Geometry check sheet. Reference: the model listing, model coordinates, mm. Face numbers are marked on the shaded views. A direction names the side the tool comes from. Give positions to 0.01 mm unless a question says otherwise; leave off trailing zeros. Use CSV: the item, a comma, the result in double quotes. Start each with the question number.
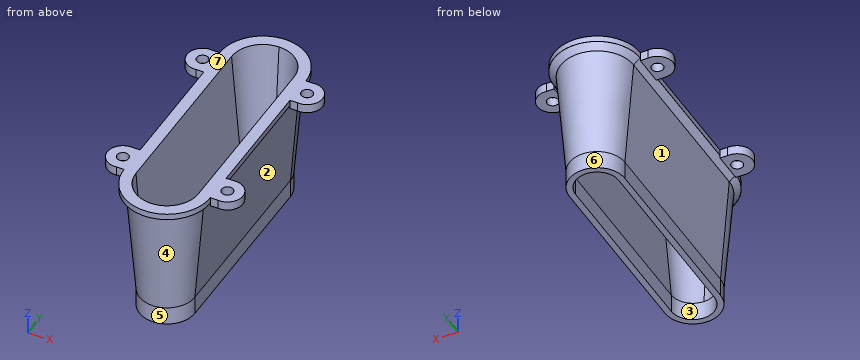
from build123d import *
from OCP.BRepFilletAPI import BRepFilletAPI_MakeChamfer

# Parameters (mm, degrees)
DODANIE_WYCI_GNI_CIE1_DEPTH  = 45
DODANIE_WYCI_GNI_CIE2_DEPTH  = 2
SFAZOWANIE1_SIZE             = 37
SFAZOWANIE1_SIZE2            = 3
SKORUPA4_DEPTH               = 45
SZKIC11_R                    = 1.9
DODANIE_WYCI_GNI_CIE11_DEPTH = 3
SFAZOWANIE6_SIZE             = 1.8
SFAZOWANIE6_SIZE2            = 1.965251773


with BuildPart() as part:
    # Szkic1 → Dodanie-wyciągnięcie1 (new body)
    with BuildSketch(Plane.XY):
        with BuildLine():
            Line((-9, 0), (-9, 60))
            ThreePointArc((-9, 60), (0, 69), (9, 60))
            Line((9, 60), (9, 0))
            ThreePointArc((9, 0), (0, -9), (-9, 0))
        make_face()
    extrude(amount=DODANIE_WYCI_GNI_CIE1_DEPTH)

    # Szkic2 → Dodanie-wyciągnięcie2 (add)
    with BuildSketch(Plane.XY.offset(45)):
        with BuildLine():
            Line((14, 60), (14, 0))
            ThreePointArc((14, 0), (0, -14), (-14, 0))
            Line((-14, 0), (-14, 60))
            ThreePointArc((-14, 60), (0, 74), (14, 60))
        make_face()
    extrude(amount=-DODANIE_WYCI_GNI_CIE2_DEPTH)

    # Sfazowanie1: one chamfer whose edges measure the first distance from different faces: ONE call of the kernel's chamfer builder (chamfer() names one face for all edges)
    sfazowanie1_edges_1 = [part.edges().sort_by_distance(p)[0] for p in [
        (-9, 30, 43),
    ]]
    sfazowanie1_side_1 = [part.faces().sort_by_distance(p)[0] for p in [
        (-9, 30, 21.5),
    ]]
    sfazowanie1_edges_2 = [part.edges().sort_by_distance(p)[0] for p in [
        (0, -9, 43),
    ]]
    sfazowanie1_side_2 = [part.faces().sort_by_distance(p)[0] for p in [
        (0, -9, 21.5),
    ]]
    sfazowanie1_edges_3 = [part.edges().sort_by_distance(p)[0] for p in [
        (9, 30, 43),
    ]]
    sfazowanie1_side_3 = [part.faces().sort_by_distance(p)[0] for p in [
        (9, 30, 21.5),
    ]]
    sfazowanie1_edges_4 = [part.edges().sort_by_distance(p)[0] for p in [
        (0, 69, 43),
    ]]
    sfazowanie1_side_4 = [part.faces().sort_by_distance(p)[0] for p in [
        (0, 69, 21.5),
    ]]
    sfazowanie1 = BRepFilletAPI_MakeChamfer(part.part.solid().wrapped)
    for e in sfazowanie1_edges_1:
        sfazowanie1.Add(SFAZOWANIE1_SIZE, SFAZOWANIE1_SIZE2, e.wrapped, sfazowanie1_side_1[0].wrapped)  # the first distance lies on this face
    for e in sfazowanie1_edges_2:
        sfazowanie1.Add(SFAZOWANIE1_SIZE, SFAZOWANIE1_SIZE2, e.wrapped, sfazowanie1_side_2[0].wrapped)  # the first distance lies on this face
    for e in sfazowanie1_edges_3:
        sfazowanie1.Add(SFAZOWANIE1_SIZE, SFAZOWANIE1_SIZE2, e.wrapped, sfazowanie1_side_3[0].wrapped)  # the first distance lies on this face
    for e in sfazowanie1_edges_4:
        sfazowanie1.Add(SFAZOWANIE1_SIZE, SFAZOWANIE1_SIZE2, e.wrapped, sfazowanie1_side_4[0].wrapped)  # the first distance lies on this face
    add(Compound.cast(sfazowanie1.Shape()), mode=Mode.REPLACE)

    # Skorupa4: read off the stored shape, not the designer's step
    # Skorupa4 outline → Skorupa4 (cut)
    with BuildSketch(Plane.XY):
        with BuildLine():
            ThreePointArc((-7, 0), (0, -7), (7, 0))
            Line((7, 0), (7, 60))
            ThreePointArc((7, 60), (0, 67), (-7, 60))
            Line((-7, 60), (-7, 0))
        make_face()
    extrude(amount=SKORUPA4_DEPTH, mode=Mode.SUBTRACT)

    # Skorupa4 2: loft between two sections, ruled curve by curve
    skorupa4_2_from = [
        Edge.make_three_point_arc((7, 60, 6.080948258), (4.949747468, 64.949747468, 6.080948258), (0, 67, 6.080948258)),
        Edge.make_three_point_arc((0, 67, 6.080948258), (-4.949747468, 64.949747468, 6.080948258), (-7, 60, 6.080948258)),
        Edge.make_three_point_arc((-7, 0, 6.080948258), (-4.949747468, -4.949747468, 6.080948258), (0, -7, 6.080948258)),
        Edge.make_three_point_arc((0, -7, 6.080948258), (4.949747468, -4.949747468, 6.080948258), (7, 0, 6.080948258)),
        Edge.make_line((7, 0, 6.080948258), (7, 60, 6.080948258)),
        Edge.make_line((-7, 60, 6.080948258), (-7, 0, 6.080948258)),
    ]
    skorupa4_2_to = [
        Edge.make_three_point_arc((10.15559879, 60, 45), (7.181092771, 67.181092771, 45), (0, 70.15559879, 45)),
        Edge.make_three_point_arc((0, 70.15559879, 45), (-7.181092771, 67.181092771, 45), (-10.15559879, 60, 45)),
        Edge.make_three_point_arc((-10.15559879, 0, 45), (-7.181092771, -7.181092771, 45), (0, -10.15559879, 45)),
        Edge.make_three_point_arc((0, -10.15559879, 45), (7.181092771, -7.181092771, 45), (10.15559879, 0, 45)),
        Edge.make_line((10.15559879, 0, 45), (10.15559879, 60, 45)),
        Edge.make_line((-10.15559879, 60, 45), (-10.15559879, 0, 45)),
    ]
    skorupa4_2 = Solid(Shell([*[Face.make_surface_from_curves(skorupa4_2_from[k], skorupa4_2_to[k]) for k in range(6)], Face(Wire(skorupa4_2_from)), Face(Wire(skorupa4_2_to))]))
    add(skorupa4_2, mode=Mode.SUBTRACT)

    # Szkic11 → Dodanie-wyciągnięcie11 (add)
    # profile 1 of 4: a face of its own
    with BuildSketch(Plane.XY.offset(45)):
        with BuildLine():
            Line((14, 0), (16.5, 0))
            ThreePointArc((16.5, 0), (22.024937811, 5), (16.5, 10))
            Line((16.5, 10), (14, 10))
            Line((14, 10), (14, 0))
        make_face()
        with Locations((17, 5)):
            Circle(SZKIC11_R, mode=Mode.SUBTRACT)
    # profile 2 of 4: a face of its own
    with BuildSketch(Plane.XY.offset(45)):
        with BuildLine():
            Line((-14, 10), (-16.5, 10))
            ThreePointArc((-16.5, 10), (-22.024937811, 5), (-16.5, 0))
            Line((-16.5, 0), (-14, 0))
            Line((-14, 0), (-14, 10))
        make_face()
        with Locations(Location((-17, 5, 0), (0, 0, 180))):
            Circle(SZKIC11_R, mode=Mode.SUBTRACT)
    # profile 3 of 4: a face of its own
    with BuildSketch(Plane.XY.offset(45)):
        with BuildLine():
            Line((-14, 60), (-16.5, 60))
            ThreePointArc((-16.5, 60), (-22.024937811, 55), (-16.5, 50))
            Line((-16.5, 50), (-14, 50))
            Line((-14, 50), (-14, 60))
        make_face()
        with Locations((-17, 55)):
            Circle(SZKIC11_R, mode=Mode.SUBTRACT)
    # profile 4 of 4: a face of its own
    with BuildSketch(Plane.XY.offset(45)):
        with BuildLine():
            Line((14, 50), (16.5, 50))
            ThreePointArc((16.5, 50), (22.024937811, 55), (16.5, 60))
            Line((16.5, 60), (14, 60))
            Line((14, 60), (14, 50))
        make_face()
        with Locations(Location((17, 55, 0), (0, 0, 180))):
            Circle(SZKIC11_R, mode=Mode.SUBTRACT)
    extrude(amount=-DODANIE_WYCI_GNI_CIE11_DEPTH)

    # Sfazowanie6: one chamfer whose edges measure the first distance from different faces: ONE call of the kernel's chamfer builder (chamfer() names one face for all edges)
    sfazowanie6_edges_1 = [part.edges().sort_by_distance(p)[0] for p in [
        (12, 30, 43),
    ]]
    sfazowanie6_side_1 = [part.faces().sort_by_distance(p)[0] for p in [
        (10.5, 30, 24.5),
    ]]
    sfazowanie6_edges_2 = [part.edges().sort_by_distance(p)[0] for p in [
        (0, 72, 43),
    ]]
    sfazowanie6_side_2 = [part.faces().sort_by_distance(p)[0] for p in [
        (0, 70.5, 24.5),
    ]]
    sfazowanie6_edges_3 = [part.edges().sort_by_distance(p)[0] for p in [
        (0, -12, 43),
    ]]
    sfazowanie6_side_3 = [part.faces().sort_by_distance(p)[0] for p in [
        (0, -10.5, 24.5),
    ]]
    sfazowanie6_edges_4 = [part.edges().sort_by_distance(p)[0] for p in [
        (-12, 30, 43),
    ]]
    sfazowanie6_side_4 = [part.faces().sort_by_distance(p)[0] for p in [
        (-10.5, 30, 24.5),
    ]]
    sfazowanie6 = BRepFilletAPI_MakeChamfer(part.part.solid().wrapped)
    for e in sfazowanie6_edges_1:
        sfazowanie6.Add(SFAZOWANIE6_SIZE, SFAZOWANIE6_SIZE2, e.wrapped, sfazowanie6_side_1[0].wrapped)  # the first distance lies on this face
    for e in sfazowanie6_edges_2:
        sfazowanie6.Add(SFAZOWANIE6_SIZE, SFAZOWANIE6_SIZE2, e.wrapped, sfazowanie6_side_2[0].wrapped)  # the first distance lies on this face
    for e in sfazowanie6_edges_3:
        sfazowanie6.Add(SFAZOWANIE6_SIZE, SFAZOWANIE6_SIZE2, e.wrapped, sfazowanie6_side_3[0].wrapped)  # the first distance lies on this face
    for e in sfazowanie6_edges_4:
        sfazowanie6.Add(SFAZOWANIE6_SIZE, SFAZOWANIE6_SIZE2, e.wrapped, sfazowanie6_side_4[0].wrapped)  # the first distance lies on this face
    add(Compound.cast(sfazowanie6.Shape()), mode=Mode.REPLACE)


solid = part.part
(1) Draft check along X on the marked faces 1, 2, 3 and 4. Enter one of: +X half, -X half, draft (parallel to the pull), parting line (faces both ways), or undercut.
(2) Sectioned sample at A-A on y = 5. Give the number of separate pieces and of enclosed holes in the cut face, then the cut area to 3 significant figures.
(3) Go/stop test with flat-tipped pins: P1, Ø2, axis at x = -15.5, z = 43, coming from the -Y side; P2, Ø6, axis at x = 1.5, y = 37, coming from the -Z side; P3, Ø8, axis at x = 9, z = 10, coming from the -Y side; P4, Ø5, axis at x = -17, y = 55, coming from the -Z side. Record where each tip stops, or that it passes through.
(4) Thickness scan on line 1 (Y direction, x = -17, z = 43); line 2 (X direction, y = 7, z = 6); line 3 (X direction, y = 17.5, z = 19). Record the ranges inside material, lowest first.
(5) Access from +Z, -Z, +X, -X, +Y, -Y to the whole of each face (thin tool, end or side, straight path). Record for the marked faces 5, 6 and 7.
Responses:
1,face 1,"-X half"
1,face 2,"+X half"
1,face 3,"undercut"
1,face 4,"parting line"
2,separate pieces,"4"
2,enclosed holes,"0"
2,area,"217 mm2"
3,P1,"y = 0"
3,P2,"through"
3,P3,"y = -7.9"
3,P4,"z = 42"
4,line 1,"-0.02 to 3.1, 6.9 to 10.02, 49.98 to 53.1, 56.9 to 60.02"
4,line 2,"-9 to -7, 7 to 9"
4,line 3,"-10.05 to -8.05, 8.05 to 10.05"
5,face 5,"-Z, -Y"
5,face 6,"-Z, +Y"
5,face 7,"+Z, +X, -X, +Y, -Y"
